Geometry: final body of the model. Coordinates: model frame, mm. Coordinates: 2 decimals unless noted, no trailing zeros. Write each loop counter-clockwise with the first axis right and the second up, starting at its lowest first coordinate (ties: lowest second). Pieces come first, ordered by that corner, then holes. Notation, with made-up numbers: (11, 63) -> (49, 63) arc R21 ccw to (49, 82) -> close; hole circle Ø9 at (76, -8). An arc over 180 degrees is marked (long way). One line per item, written item: value.
```python
from build123d import *

# Parameters (mm, degrees)
CYLINDER_R             = 12.7
CYLINDER_DEPTH         = 539.75
CYLINDER_ROLL_ANGLE    = 90
BASEFEATURE_ROLL_ANGLE = -90
SKETCH_R               = 2.54
POCKET_DEPTH           = 25.401
BODY_ROLL_ANGLE        = 90


with BuildPart() as part:
    # Cylinder → Cylinder (new body)
    with BuildSketch(Plane.XY):
        Circle(CYLINDER_R)
    extrude(amount=CYLINDER_DEPTH)


with BuildPart() as part_1:
    # Cylinder roll: moved
    add(part.part.rotate(Axis((0, 0, 0), (1, 0, 0)), CYLINDER_ROLL_ANGLE))


with BuildPart() as part_2:
    # Cylinder placement: moved
    add(part_1.part)


with BuildPart() as part_3:
    # BaseFeature roll: moved
    add(part_2.part.rotate(Axis((0, 0, 0), (1, 0, 0)), BASEFEATURE_ROLL_ANGLE))


with BuildPart() as part_4:
    # BaseFeature placement: moved
    add(part_3.part)

    # Sketch (on DatumPlane) → Pocket (cut, through all)
    with BuildSketch(Plane(origin=(12.7, 0, 269.875), x_dir=(0, -1, 0), z_dir=(1, 0, 0))):
        with Locations((0, -257.175)):
            Circle(SKETCH_R)
        with Locations((0, 257.175)):
            Circle(SKETCH_R)
    extrude(amount=-POCKET_DEPTH, mode=Mode.SUBTRACT)


with BuildPart() as part_5:
    # Body roll: moved
    add(part_4.part.rotate(Axis((0, 0, 0), (1, 0, 0)), BODY_ROLL_ANGLE))


with BuildPart() as part_6:
    # Body placement: moved
    add(part_5.part)


solid = part_6.part
```
(1) First-contact query: pin 1 (4.5 mm diameter, centred on y = -527.05, z = 0, fed in from -X); pin 2 (1 mm diameter, centred on y = -480, z = -8, fed in from +X); pin 3 (5 mm diameter, centred on x = -8.5, y = -75, fed in from +Z); pin 4 (6 mm diameter, centred on y = -405, z = -5, fed in from +X). Flat tips, straight axial feed; report the tip coordinate or a pass-through.
Responses:
pin 1: passes through
pin 2: stops at x = 10.25
pin 3: stops at z = 11.19
pin 4: stops at x = 12.54
(2) Line query: line 1 (Y direction, x = -6, z = 0); line 2 (Z direction, x = -1.5, y = -274); line 3 (Z direction, x = 0, y = -196.5). Output: solid intervals per line, ascending. Write a range as [from, to].
Responses:
line 1: y = [-539.75, -529.59], [-524.51, -15.24], [-10.16, 0]
line 2: z = [-12.61, 12.61]
line 3: z = [-12.7, 12.7]
(3) Section B-B (y = -432.5). Return the cut outline in (x, z), then the cut area to 3 significant figures.
Responses:
outline: circle Ø25.4 at (0, 0)
area: 507 mm2
(4) Section A-A (x = 3.5). Return the cut outline in (y, z), then the cut area to 3 significant figures.
Responses:
outline: (-539.75, -12.21) -> (0, -12.21) -> (0, 12.21) -> (-539.75, 12.21) -> close; hole circle Ø5.08 at (-527.05, 0); hole circle Ø5.08 at (-12.7, 0)
area: 13,100 mm2
